Autodesk Inventor part; units mm, degrees
ref_plane "YZ Plane" through (0, 0, 0) normal (1, 0, 0) x (0, 1, 0)
ref_plane "XZ Plane" through (0, 0, 0) normal (0, 1, 0) x (-1, 0, 0)
ref_plane "XY Plane" through (0, 0, 0) normal (0, 0, 1) x (1, 0, 0)
sketch "Sketch1" plane through (0, 0, 0) normal (0, 1, 0) x (-1, 0, 0)
  line L0 (-20, 40) -> (20, 40)
  line L1 (20, 40) -> (20, -40)
  line L2 (20, -40) -> (-20, -40)
  line L3 (-20, -40) -> (-20, 40)
  line L4 (-20, 40) -> (20, -40) construction
  line L5 (20, 40) -> (-20, -40) construction
  line L6 (-17.76, 37.76) -> (17.76, 37.76)
  line L7 (17.76, 37.76) -> (17.76, -37.76)
  line L8 (17.76, -37.76) -> (-17.76, -37.76)
  line L9 (-17.76, -37.76) -> (-17.76, 37.76)
  line L10 (-17.76, 37.76) -> (17.76, -37.76) construction
  line L11 (17.76, 37.76) -> (-17.76, -37.76) construction
  point P0 (0, 0)
  dimension "d0" = 40
  dimension "d1" = 80
  dimension "d2" = 35.52
  dimension "d10" = 2.24
extrude "Extrusion1" add sketch "Sketch1" along normal blind 1824.7
fillet "Fillet1" radius 2 4 edges at (-17.76, 912.35, 37.76) (17.76, 912.35, -37.76) (17.76, 912.35, 37.76) (-17.76, 912.35, -37.76)
fillet "Fillet1" radius 4 4 edges at (20, 912.35, 40) (-20, 912.35, 40) (20, 912.35, -40) (-20, 912.35, -40)
sketch "Boceto3" plane through (-16, 0, 40) normal (0, 0, 1) x (1, 0, 0)
  circle A0 centre (16, 11.25) radius 4.5
  circle A1 centre (16, 68.75) radius 4.5
  circle A2 centre (16, 911.25) radius 4.5
  circle A3 centre (16, 968.75) radius 4.5
  circle A4 centre (16, 1268.75) radius 4.5
  circle A5 centre (16, 1211.25) radius 4.5
  circle A6 centre (16, 968.75) radius 5.5
  circle A7 centre (16, 911.25) radius 5.5
  circle A8 centre (16, 68.75) radius 5.5
  circle A9 centre (16, 11.25) radius 5.5
  circle A10 centre (16, 1268.75) radius 5.5
  circle A11 centre (16, 1211.25) radius 5.5
  point P0 (16, 0)
  dimension "d11" = 11
  dimension "d12" = 11
  dimension "d13" = 11
  dimension "d14" = 11
  dimension "d15" = 11
  dimension "d16" = 11
extrude "Extrusión3" cut sketch "Boceto3" against normal blind 10 contours A0 | A1 | A2 | A3 | A4 | A5 | A6 | A7 | A8 | A9 | A10 | A11
sketch "Sketch8" plane through (20, 0, 36) normal (1, 0, 0) x (0, 0, -1)
  circle A0 centre (47.8654, 1771.4414) radius 11.11
  point P0 (36, 0)
extrude "Extrusion7" cut sketch "Sketch8" against normal through all
sketch "Sketch12" plane through (20, 0, 36) normal (1, 0, 0) x (0, 0, -1)
  line L0 (76, 1824.7) -> (76, 0)
  line L1 (76, 0) -> (17, 0)
  line L2 (0, 0) -> (72, 0)
  line L3 (17, 0) -> (17, 35)
  line L4 (17, 0) -> (17, 555)
  line L5 (17, 0) -> (17, 1095)
  line L6 (17, 0) -> (17, 1615)
  point P0 (36, 0)
  dimension "d37" = 59
  dimension "d38" = 35
  dimension "d39" = 555
  dimension "d40" = 1095
  dimension "d41" = 1615
hole "Hole1" at (20, 35, 19) at (20, 555, 19) at (20, 1095, 19) at (20, 1615, 19) direction (-1, 0, 0) diameter 4.5 depth 8 tip angle 118
sketch "Sketch13" plane through (20, 0, 36) normal (1, 0, 0) x (0, 0, -1)
  circle A0 centre (54.5, 11.25) radius 3.3234
  circle A1 centre (54.5, 68.75) radius 3.3234
  point P0 (36, 0)
hole "Hole2" at (20, 11.25, -18.5) at (20, 68.75, -18.5) direction (-1, 0, 0) diameter 11 depth 8
sketch "Sketch15" plane through (-16, 0, -40) normal (0, 0, -1) x (-1, 0, 0)
  line L0 (-10, 0) -> (-10, 80)
  line L1 (-10, 0) -> (70, 0) construction
  line L2 (4, 0) -> (4, 1824.7) construction
  line L3 (4, 80) -> (-32.0092, 80) construction
  line L4 (-10, 80) -> (-10, 1664.7)
  line L5 (-10, 872.35) -> (-10, 1572.35)
  line L6 (-10, 872.35) -> (-5, 872.35)
  point P0 (-16, 0)
  point P1 (-10, 172.35)
  dimension "d56" = 80
  dimension "d57" = 90
  dimension "d58" = 14
  dimension "d59" = 700
  dimension "d60" = 5
  dimension "d68" = 792.35
hole "Hole3" at (-6, 172.35, -40) at (-6, 872.35, -40) at (-6, 1572.35, -40) direction (0, 0, 1) diameter 4.5 depth 8
properties part number "SP43V1 Tubo 40x80x1825mm" material "Acero, carbono"
Geometry: final body of the model. Coordinates: model frame, mm. A direction names the side the tool comes from. Give positions to 0.01 mm unless a question says otherwise; leave off trailing zeros. Order: outer loops, then holes, each group sorted by start corner. A loop starts at its lowest first (then second) coordinate and runs counter-clockwise, first axis right, second up. Notation, with made-up numbers: (40, 10) - (64, 10) arc R14 cw to (64, 35) - close; hole circle Ø2 at (55, 9.5). An arc over 180 degrees is marked (long way). Use CSV: the item, a comma, the result in double quotes.
1. Section query A-A (y = 506). Output: boundary loops of the cut face in (x, z), plus the area to 3 significant figures.
Answers below:
outline,"(-20, -36) arc R4 ccw to (-16, -40) - (16, -40) arc R4 ccw to (20, -36) - (20, 36) arc R4 ccw to (16, 40) - (-16, 40) arc R4 ccw to (-20, 36) - close; hole (-17.76, -35.76) arc R2 ccw to (-15.76, -37.76) - (15.76, -37.76) arc R2 ccw to (17.76, -35.76) - (17.76, 35.76) arc R2 ccw to (15.76, 37.76) - (-15.76, 37.76) arc R2 ccw to (-17.76, 35.76) - close"
area,"507 mm2"
2. Access query for faces 1 (the face through (0, 900, -40)), 2 (the face through (0, 900, -37.76)). Directions: +Z, -Z, +X, -X, +Y, -Y. A direction counts if a zero-diameter tool reaches every point of the face in a straight line with its end or side. Return the directions, or none.
Answers below:
face 1,"-Z, +X, -X, +Y, -Y"
face 2,"+Y, -Y"
3. Mould query, pull axis X, two halves, no side actions, for faces 3 (the face through (-20, 900, 1)), 4 (the face through (20, 900, -1)), 5 (the face through (0, 900, 37.76)), 6 (the face through (0, 900, 40)). Classes: +X half, -X half, draft (parallel to the pull), parting line (faces both ways), or undercut.
Answers below:
face 3,"-X half"
face 4,"+X half"
face 5,"undercut"
face 6,"draft"
4. Material intervals for line 1 along Y through (x, z) = (-6, -38.3); line 2 along Y through (x, z) = (19.2, 19); line 3 along Z through (x, y) = (-7, 1047.5), sorted ascending. Write a range as from..to.
Answers below:
line 1,"0..170.1, 174.6..870.1, 874.6..1570.1, 1574.6..1824.7"
line 2,"0..32.75, 37.25..552.75, 557.25..1092.75, 1097.25..1612.75, 1617.25..1824.7"
line 3,"-40..-37.76, 37.76..40"
